Geometry check sheet. Reference: the model listing, model coordinates, mm. A direction names the side the tool comes from. Round coordinates to 2 decimals unless told otherwise and drop trailing zeros. Order: outer loops, then holes, each group sorted by start corner. A loop starts at its lowest first (then second) coordinate and runs counter-clockwise, first axis right, second up. Notation, with made-up numbers: (50, 77.5) -> (87, 77.5) arc R15 ccw to (87, 104.5) -> close; hole circle Ø5 at (32, -12.75). An arc over 180 degrees is marked (long way). Use a Markdown table: item, result. Add a question column.
Item 1: Sectioned sample at A-A, the plane z = -1. Record the cut outline in (x, y).
Item 2: Mould release check, pull along X, two halves, no side actions. Record for faces 1 (the flat face through (-27.616, -318, 0)), 2 (the flat face through (12, -318, -12.759)), 3 (the flat face through (-33.616, -318, -3)), 4 (the flat face through (54.384, -318, 0)): pulls with the +X half, pulls with the -X half, needs draft (parallel to the pull), parting line crosses it, or undercut.
Item 3: Material ranges on probe 1 along X at (y, z) = (-375, -5.5), recorded low to high. Write a range as [from, to].
Item 4: Sectioned sample at B-B, the plane y = -91. Record the cut outline in (x, z).
Item 5: Gauge pin test, flat end, axial feed: pin 1 Ø1.2 at (x, y) = (-30.5, -276) entering from +Z. Record the tip position at first contact, or that the pin passes through.
Item 6: Set-up check for faces 5 (the flat face through (50.384, -318, 0)), 6 (the flat face through (11, -675, -3)): record each of +Z, -Z, +X, -X, +Y, -Y from which the full face is reachable in a straight line by a thin tool's end or side.
from build123d import *

# Parameters (mm, degrees)
EXTRUDE_1_DEPTH      = 50
EXTRUDE_1_DEPTH_BACK = 675


with BuildPart() as part:
    # Эскиз1 → Бобышка-Вытянуть1 (new, two sides: drawn at the far end of the back side and taken through both)
    with BuildSketch(Plane(origin=(0, 0, 0), x_dir=(1, 0, 0), z_dir=(0, 1, 0)).offset(-EXTRUDE_1_DEPTH_BACK)):
        Polygon((-31.616298812, -7.241086587), (-31.616298812, 7.758913413), (-27.616298812, 7.758913413), (-27.616298812, -7.241086587), (50.383701188, -7.241086587), (50.383701188, 7.758913413), (54.383701188, 7.758913413), (54.383701188, -7.241086587), (56.383701188, -7.241086587), (56.383701188, 12.758913413), (-33.616298812, 12.758913413), (-33.616298812, -7.241086587), align=None)
    extrude(amount=EXTRUDE_1_DEPTH + EXTRUDE_1_DEPTH_BACK)


solid = part.part
Found:
| question | item | result |
|---|---|---|
| 1 | outline | (-33.62, -675) -> (-31.62, -675) -> (-31.62, 50) -> (-33.62, 50) -> close; (-27.62, -675) -> (50.38, -675) -> (50.38, 50) -> (-27.62, 50) -> close; (54.38, -675) -> (56.38, -675) -> (56.38, 50) -> (54.38, 50) -> close |
| 2 | face 1 | undercut |
| 2 | face 2 | needs draft |
| 2 | face 3 | pulls with the -X half |
| 2 | face 4 | undercut |
| 3 | probe 1 | x = [-33.62, -31.62], [-27.62, 50.38], [54.38, 56.38] |
| 4 | outline | (-33.62, -12.76) -> (56.38, -12.76) -> (56.38, 7.24) -> (54.38, 7.24) -> (54.38, -7.76) -> (50.38, -7.76) -> (50.38, 7.24) -> (-27.62, 7.24) -> (-27.62, -7.76) -> (-31.62, -7.76) -> (-31.62, 7.24) -> (-33.62, 7.24) -> close |
| 5 | pin 1 | stops at z = -7.76 |
| 6 | face 5 | +Z, +Y, -Y |
| 6 | face 6 | +Z, -Z, +X, -X, -Y |
